from build123d import *

# Parameters (mm, degrees)
SKETCH1_W           = 85
SKETCH1_H           = 51
SKETCH1_R           = 13.75
SKETCH1_R_2         = 2.25
BOSS_EXTRUDE1_DEPTH = 3.175


with BuildPart() as part:
    # Sketch1 → Boss-Extrude1 (new body)
    with BuildSketch(Plane.XY):
        Rectangle(SKETCH1_W, SKETCH1_H)
        Circle(SKETCH1_R, mode=Mode.SUBTRACT)
        with Locations((0, 17.5)):
            Circle(SKETCH1_R_2, mode=Mode.SUBTRACT)
        with Locations((17.5, 0)):
            Circle(SKETCH1_R_2, mode=Mode.SUBTRACT)
        with Locations((0, -17.5)):
            Circle(SKETCH1_R_2, mode=Mode.SUBTRACT)
        with Locations((-17.5, 0)):
            Circle(SKETCH1_R_2, mode=Mode.SUBTRACT)
        with BuildLine():
            Line((-37.5, 19.25), (-32.5, 19.25))
            ThreePointArc((-32.5, 19.25), (-30.75, 17.5), (-32.5, 15.75))
            Line((-32.5, 15.75), (-37.5, 15.75))
            ThreePointArc((-37.5, 15.75), (-39.25, 17.5), (-37.5, 19.25))
        make_face(mode=Mode.SUBTRACT)
        with BuildLine():
            Line((37.5, 19.25), (32.5, 19.25))
            ThreePointArc((32.5, 19.25), (30.75, 17.5), (32.5, 15.75))
            Line((32.5, 15.75), (37.5, 15.75))
            ThreePointArc((37.5, 15.75), (39.25, 17.5), (37.5, 19.25))
        make_face(mode=Mode.SUBTRACT)
        with BuildLine():
            Line((37.5, -19.25), (32.5, -19.25))
            ThreePointArc((32.5, -19.25), (30.75, -17.5), (32.5, -15.75))
            Line((32.5, -15.75), (37.5, -15.75))
            ThreePointArc((37.5, -15.75), (39.25, -17.5), (37.5, -19.25))
        make_face(mode=Mode.SUBTRACT)
        with BuildLine():
            Line((-37.5, -19.25), (-32.5, -19.25))
            ThreePointArc((-32.5, -19.25), (-30.75, -17.5), (-32.5, -15.75))
            Line((-32.5, -15.75), (-37.5, -15.75))
            ThreePointArc((-37.5, -15.75), (-39.25, -17.5), (-37.5, -19.25))
        make_face(mode=Mode.SUBTRACT)
    extrude(amount=BOSS_EXTRUDE1_DEPTH)


solid = part.part
The model under review builds one solid part; all positions refer to its coordinate system, in mm. A direction names the side the tool comes from. Give positions to 0.01 mm unless a question says otherwise; leave off trailing zeros. Write each loop counter-clockwise with the first axis right and the second up, starting at its lowest first coordinate (ties: lowest second). Pieces come first, ordered by that corner, then holes.
1. Tool access review of faces 1 (the flat face through (-10, 12, 3.175)), 2 (the cylindrical face through (39.25, 17.46, 1.57)): name each direction out of +Z, -Z, +X, -X, +Y, -Y from which nothing blocks a thin tool from reaching the whole face with its end or side.
2. Add section C-C, the plane z = 0.6. Count the separate pieces of the cut face and the enclosed holes in it, plus the area to 3 significant figures.
3. Add section B-B, the plane x = 17.5. Write out the cut boundary in (y, z) (3 decimals), plus the area to 3 significant figures.
4. Draft analysis for pull direction X (two halves, no side actions). For faces 3 (the flat face through (-10, 12, 0)), 4 (the flat face through (-35, -15.75, 2)), 5 (the flat face through (-42.5, 0, 2)), 6 (the flat face through (-35, -19.25, 2)), state which applies: +X half, -X half, draft (parallel to the pull), parting line (faces both ways), or undercut.
5. For P1, Ø2.5, axis at x = 0, y = -17.5, coming from the -Z side, flat-tipped, find the tip position at first contact; note if it passes through.
6. Add section A-A, the plane y = -17.5. Write out the cut boundary in (x, z) (3 decimals).
7. Wall thickness on L1, parallel to Y at x = 0, z = 2; L2, parallel to Y at x = -17.5, z = 1.7; L3, parallel to Y at x = -32, z = 2.1: over which ranges is each line inside the solid? List them lowest first.
Worked answers:
1. face 1: +Z, +X, -X, +Y, -Y
1. face 2: +Z, -Z
2. separate pieces: 1
2. enclosed holes: 9
2. area: 3,570 mm2
3. outline: (-25.5, 0) - (-2.25, 0) - (-2.25, 3.175) - (-25.5, 3.175) - close; (2.25, 0) - (25.5, 0) - (25.5, 3.175) - (2.25, 3.175) - close
3. area: 148 mm2
4. face 3: draft
4. face 4: undercut
4. face 5: -X half
4. face 6: undercut
5. P1: passes through
6. outline: (-42.5, 0) - (-39.25, 0) - (-39.25, 3.175) - (-42.5, 3.175) - close; (-30.75, 0) - (-2.25, 0) - (-2.25, 3.175) - (-30.75, 3.175) - close; (2.25, 0) - (30.75, 0) - (30.75, 3.175) - (2.25, 3.175) - close; (39.25, 0) - (42.5, 0) - (42.5, 3.175) - (39.25, 3.175) - close
7. L1: y = -25.5 to -19.75, -15.25 to -13.75, 13.75 to 15.25, 19.75 to 25.5
7. L2: y = -25.5 to -2.25, 2.25 to 25.5
7. L3: y = -25.5 to -19.18, -15.82 to 15.82, 19.18 to 25.5
